Check sheet for the drawn part. Datum: minimum x, y, z corner. Units: mm. A direction names the side the tool comes from. Give positions to 0.01 mm unless a question says otherwise; leave off trailing zeros. Order: outer loops, then holes, each group sorted by start corner. A loop starts at its lowest first (then second) coordinate and runs counter-clockwise, first axis right, second up. Notation, with made-up numbers: M -25,6 L 27,6 A15 ccw 27,24 Z; hole C 48.5,43 d10. An arc over 180 degrees is marked long. Answer as CSV lines item,"result". Start each with the question number.
Q1. Section check A-A, the plane y = 62.5. Record the boundary of the cut face in (x, z), then the cut area to 3 significant figures.
Q2. Section check D-D, the plane y = 49. Record the boundary of the cut face in (x, z), then the cut area to 3 significant figures.
Q3. Section check C-C, the plane z = 44.5. Record the boundary of the cut face in (x, y), then the cut area to 3 significant figures.
Q4. Thickness scan on line 1 (Y direction, x = 29, z = 31.5); line 2 (Z direction, x = 22.5, y = 38); line 3 (Z direction, x = 6.5, y = 62). Record the ranges inside material, lowest first.
Q5. Go/stop test with flat-tipped pins: pin 1 (4.5 mm diameter, centred on x = 10, y = 43, fed in from +Z); pin 2 (6 mm diameter, centred on x = 23.5, z = 10, fed in from +Y); pin 3 (12 mm diameter, centred on x = 10, y = 14, fed in from +Z); pin 4 (13 mm diameter, centred on x = 11, y = 62, fed in from +Z). Record where each tip stops, or that it passes through.
Q6. Mould release check, pull along Y, two halves, no side actions. Record for the marked faces 5, 6, 7 and 8: +Y half, -Y half, draft (parallel to the pull), parting line (faces both ways), or undercut.
Q7. Section check B-B, the plane x = 23. Record the boundary of the cut face in (y, z).
Q8. Set-up check for the marked faces 1, 2, 3 and 4: record each of +Z, -Z, +X, -X, +Y, -Y from which the full face is reachable in a straight line by a thin tool's end or side.
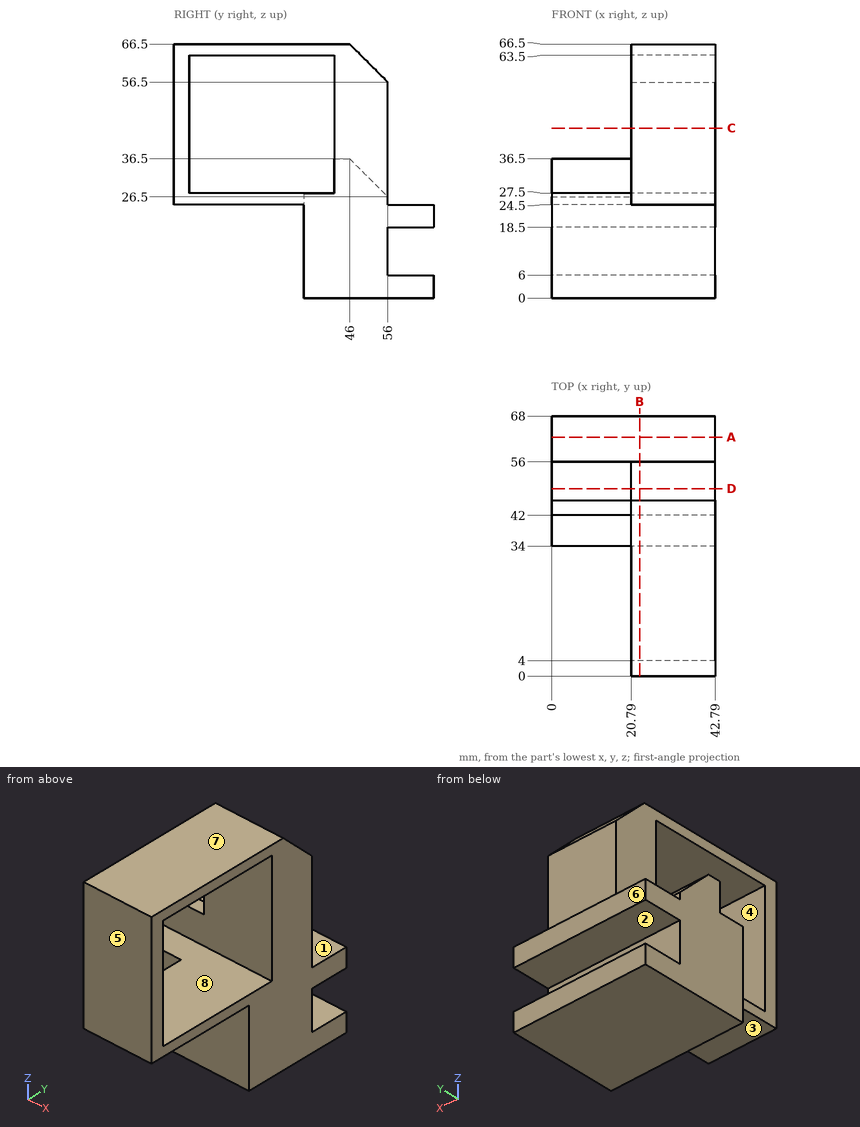
Answer block:
1,outline,"M 0,0 L 42.79,0 L 42.79,6 L 0,6 Z; M 0,18.5 L 42.79,18.5 L 42.79,24.5 L 0,24.5 Z"
1,area,"513 mm2"
2,outline,"M 0,0 L 42.79,0 L 42.79,63.5 L 20.79,63.5 L 20.79,33.5 L 0,33.5 Z"
2,area,"2,090 mm2"
3,outline,"M 20.79,0 L 42.79,0 L 42.79,4 L 20.79,4 Z; M 20.79,42 L 42.79,42 L 42.79,56 L 20.79,56 Z"
3,area,"396 mm2"
4,line 1,"y = 0 to 4, 42 to 56"
4,line 2,"z = 0 to 27.5, 63.5 to 66.5"
4,line 3,"z = 0 to 6, 18.5 to 24.5"
5,pin 1,"stops at z = 36.5"
5,pin 2,"stops at y = 56"
5,pin 3,"passes through"
5,pin 4,"stops at z = 27"
6,face 5,"-Y half"
6,face 6,"+Y half"
6,face 7,"draft"
6,face 8,"undercut"
7,outline,"M 0,24.5 L 34,24.5 L 34,0 L 68,0 L 68,6 L 56,6 L 56,18.5 L 68,18.5 L 68,24.5 L 56,24.5 L 56,56.5 L 46,66.5 L 0,66.5 Z; hole M 4,27.5 L 42,27.5 L 42,63.5 L 4,63.5 Z"
8,face 1,"+Z, +X, -X, +Y"
8,face 2,"+X, -X, +Y"
8,face 3,"-Z, +X, -X, -Y"
8,face 4,"+X, -X"
